Job drawing, mm, ordinate dimensions from the low corner. One solid piece. A direction names the side the tool comes from. Coordinates: 2 decimals unless noted, no trailing zeros. Order: outer loops, then holes, each group sorted by start corner. A loop starts at its lowest first (then second) coordinate and runs counter-clockwise, first axis right, second up. Notation, with made-up numbers: (12.5, -31.75) - (30.5, -31.75) arc R13 cw to (30.5, -10.75) - close; hole circle Ø5 at (-37.75, 75). An arc over 180 degrees is marked (long way). Return JSON: item names as keys, results as strings.
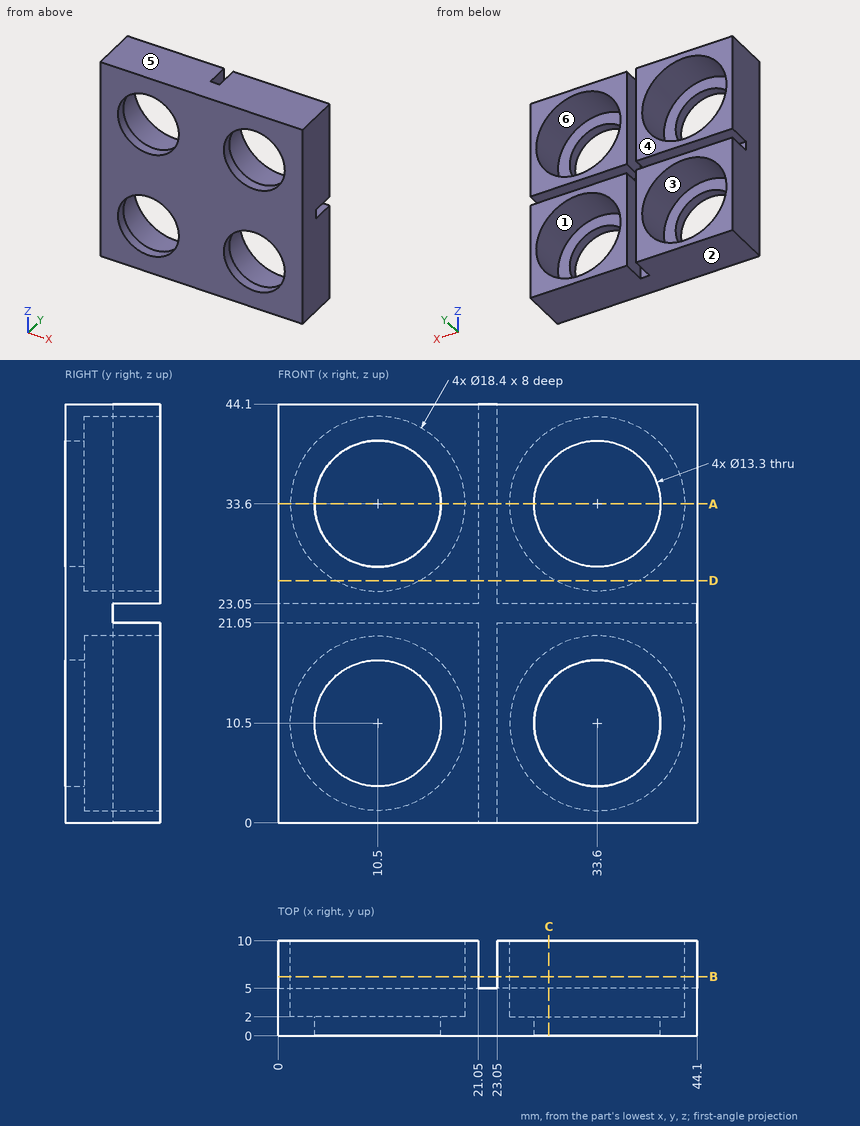
1. Drop flat-ended pins along their axis: pin 1 (16.5 mm diameter, centred on x = 33.6, z = 10.5, fed in from +Y); pin 2 (12 mm diameter, centred on x = 33.6, z = 33.6, fed in from +Y). Give the stop position or say it passes through.
Check values:
{"pin 1": "y = 2", "pin 2": "through"}
2. Cut at D-D on z = 25.5. Give the cut face in (x, y), plus the area to 3 significant figures.
Check values:
{"outline": "(0, 0) - (44.1, 0) - (44.1, 10) - (37.96, 10) - (37.96, 2) - (29.24, 2) - (29.24, 10) - (23.05, 10) - (23.05, 5) - (21.05, 5) - (21.05, 10) - (14.86, 10) - (14.86, 2) - (6.14, 2) - (6.14, 10) - (0, 10) - close", "area": "291 mm²"}
3. Mould opens along Z. For the marked faces 1, 2, 3 and 4 say: pulls with the +Z half, pulls with the -Z half, needs draft (parallel to the pull), parting line crosses it, or undercut.
Check values:
{"face 1": "undercut", "face 2": "pulls with the -Z half", "face 3": "undercut", "face 4": "needs draft"}
4. Cut at A-A on z = 33.6. Give the cut face in (x, y), plus the area to 3 significant figures.
Check values:
{"outline": "(0, 0) - (3.85, 0) - (3.85, 2) - (1.3, 2) - (1.3, 10) - (0, 10) - close; (17.15, 0) - (26.95, 0) - (26.95, 2) - (24.4, 2) - (24.4, 10) - (23.05, 10) - (23.05, 5) - (21.05, 5) - (21.05, 10) - (19.7, 10) - (19.7, 2) - (17.15, 2) - close; (40.25, 0) - (44.1, 0) - (44.1, 10) - (42.8, 10) - (42.8, 2) - (40.25, 2) - close", "area": "83.4 mm²"}
5. Cut at C-C on x = 28.5. Give the cut face in (y, z), plus the area to 3 significant figures.
Check values:
{"outline": "(0, 0) - (10, 0) - (10, 2.84) - (2, 2.84) - (2, 6.23) - (0, 6.23) - close; (0, 14.77) - (2, 14.77) - (2, 18.16) - (10, 18.16) - (10, 21.05) - (5, 21.05) - (5, 23.05) - (10, 23.05) - (10, 25.94) - (2, 25.94) - (2, 29.33) - (0, 29.33) - close; (0, 37.87) - (2, 37.87) - (2, 41.26) - (10, 41.26) - (10, 44.1) - (0, 44.1) - close", "area": "152 mm²"}
6. Tool access for the marked faces 5 and 6: list every direction of +Z, -Z, +X, -X, +Y, -Y with a clear straight run to the whole face (end or side of a thin tool).
Check values:
{"face 5": "+Z, +X, -X, +Y, -Y", "face 6": "+Y"}
7. Cut at B-B on y = 6.25. Give the cut face in (x, z).
Check values:
{"outline": "(0, 0) - (21.05, 0) - (21.05, 21.05) - (0, 21.05) - close; (0, 23.05) - (21.05, 23.05) - (21.05, 44.1) - (0, 44.1) - close; (23.05, 0) - (44.1, 0) - (44.1, 21.05) - (23.05, 21.05) - close; (23.05, 23.05) - (44.1, 23.05) - (44.1, 44.1) - (23.05, 44.1) - close; hole circle Ø18.4 at (10.5, 10.5); hole circle Ø18.4 at (10.5, 33.6); hole circle Ø18.4 at (33.6, 10.5); hole circle Ø18.4 at (33.6, 33.6)"}
8. Probe L1, parallel to X at y = 0.8, z = 33.6; L2, parallel to X at y = 4, z = 10.5; L3, parallel to Z at x = 33.6, y = 7. List the from-to ranges inside material, lowest first.
Check values:
{"L1": "0 to 3.85, 17.15 to 26.95, 40.25 to 44.1", "L2": "0 to 1.3, 19.7 to 24.4, 42.8 to 44.1", "L3": "0 to 1.3, 19.7 to 21.05, 23.05 to 24.4, 42.8 to 44.1"}
